Could you check a few things on this model? Use its own coordinates, in mm. Give positions to 0.01 mm unless a question says otherwise; leave off trailing zeros. Order: outer loops, then holes, each group sorted by start corner. A loop starts at its lowest first (then second) coordinate and runs counter-clockwise, first axis right, second up. Notation, with made-up numbers: (55, 27) - (90, 27) arc R22 ccw to (90, 53) - close; hole circle Ø3 at (-21.75, 4). An arc over 180 degrees is marked (long way). Put each result on its own line as item: value.
Autodesk Inventor part; units mm, degrees
ref_plane "YZ Plane" through (0, 0, 0) normal (1, 0, 0) x (0, 1, 0)
ref_plane "XZ Plane" through (0, 0, 0) normal (0, 1, 0) x (-1, 0, 0)
ref_plane "XY Plane" through (0, 0, 0) normal (0, 0, 1) x (1, 0, 0)
sketch "スケッチ1" plane through (0, 0, 0) normal (0, 0, 1) x (1, 0, 0)
  line L0 (0, 0) -> (10, 0)
  line L1 (10, 0) -> (10, 135)
  line L2 (10, 135) -> (0, 135)
  line L3 (0, 135) -> (0, 0)
  dimension "d0" = 10
  dimension "d1" = 135
extrude "押し出し1" add sketch "スケッチ1" along normal blind 4
sketch "スケッチ2" plane through (0, 0, 4) normal (0, 0, 1) x (1, 0, 0)
  line L0 (10, 135) -> (0, 135)
  line L1 (10, 0) -> (10, 135)
  point P0 (0, 0)
  point P1 (5, 123)
  point P2 (5, 5)
  dimension "d4" = 12
  dimension "d5" = 5
  dimension "d14" = 118
hole "穴1" at (5, 123, 4) at (5, 5, 4) direction (0, 0, -1) diameter 3.2 end through all
fillet "フィレット1" radius 2 4 edges at (0, 135, 2) (0, 0, 2) (10, 135, 2) (10, 0, 2)
properties part number "BP_BOX-Bar-add"
1) I'm going to push a flat-ended pin straight in: pin 1 (1.5 mm diameter, centred on y = 28.5, z = 1.5, fed in from -X). Where does the tip first touch, or does it pass through?
Filled in:
pin 1: stops at x = 0
2) Suppose I cut it at A-A, the plane y = 123. List the corners of the cut face in (x, z) for me, and give its area (3 significant figures).
Filled in:
outline: (0, 0) - (3.4, 0) - (3.4, 4) - (0, 4) - close; (6.6, 0) - (10, 0) - (10, 4) - (6.6, 4) - close
area: 27.2 mm^2
3) We'd pull the mould along Y, two halves only. Please class faces 1 (the flat face through (5, 0, 2)), 2 (the flat face through (5, 68, 0)), 3 (the cylindrical face through (4.93, 6.6, 1.97)): pulls with the +Y half, pulls with the -Y half, needs draft (parallel to the pull), parting line crosses it, or undercut.
Filled in:
face 1: pulls with the -Y half
face 2: needs draft
face 3: undercut
4) Suppose I cut it at B-B, the plane x = 5. List the corners of the cut face in (y, z) for me, and give its area (3 significant figures).
Filled in:
outline: (0, 0) - (3.4, 0) - (3.4, 4) - (0, 4) - close; (6.6, 0) - (121.4, 0) - (121.4, 4) - (6.6, 4) - close; (124.6, 0) - (135, 0) - (135, 4) - (124.6, 4) - close
area: 514 mm^2
5) If I drill on line 1 (Y direction, x = 5, z = 2.6); line 2 (Y direction, x = 4, z = 0.4); line 3 (X direction, y = 5, z = 2.3), over which ranges is the centre line in solid material (lowest first)? Write a range as [from, to].
Filled in:
line 1: y = [0, 3.4], [6.6, 121.4], [124.6, 135]
line 2: y = [0, 3.75], [6.25, 121.75], [124.25, 135]
line 3: x = [0, 3.4], [6.6, 10]
